Geometry: see drawing. Coordinates: mm, zero at the bounding-box minimum. Round coordinates to 2 decimals unless told otherwise and drop trailing zeros. Loops run counter-clockwise (first coordinate to the right, second up) from the corner with the lowest first, then second, coordinate; pieces in that order, holes last. Notation, with made-up numbers: M 45.5,-31 L 94.5,-31 A20 ccw 94.5,-10 Z; hole C -25,-13.5 d6. An arc over 180 degrees is marked long. Answer as a JSON object with one key per item and string values.
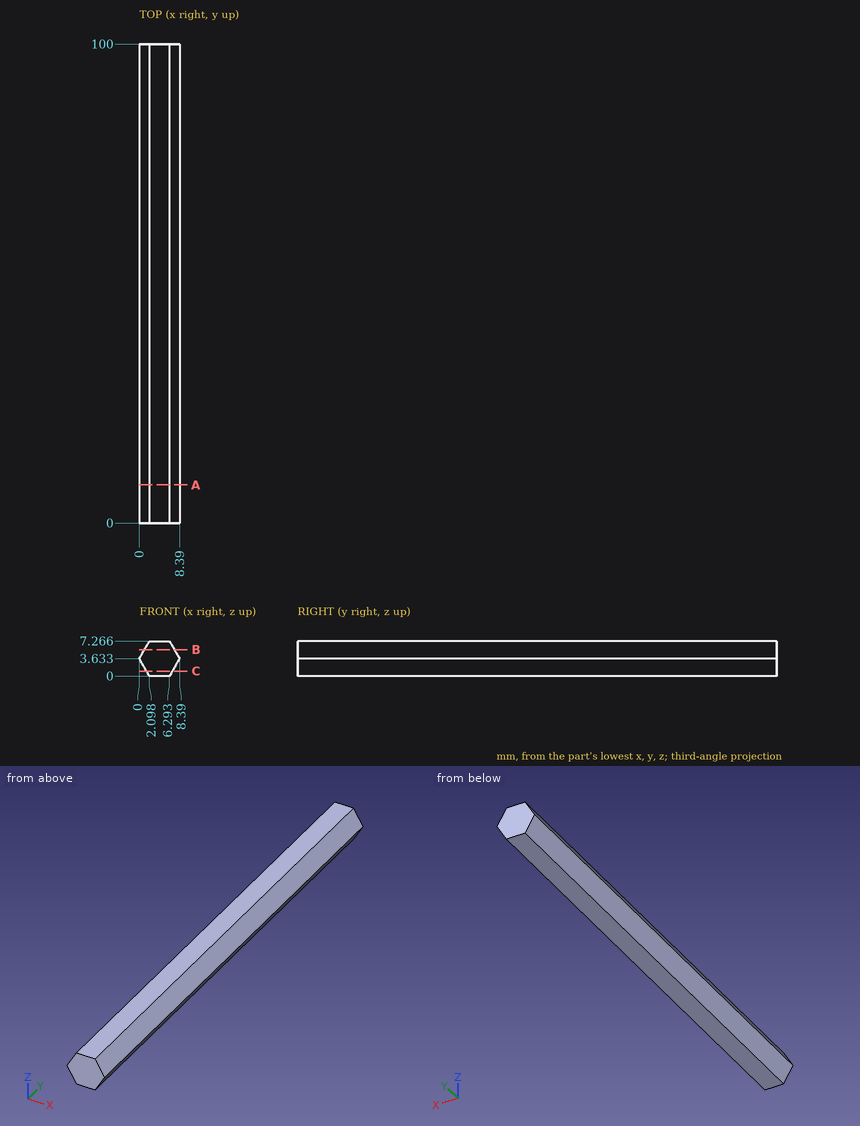
1) Pin query (flat end, axial travel): P1, Ø1, axis at y = 19.5, z = 1, coming from the -X side. Return the tip coordinate at first contact, or that it passes through.
Results:
{"P1": "x = 1.23"}
2) Section query C-C (z = 1). Return the cut outline in (x, y).
Results:
{"outline": "M 1.52,0 L 6.87,0 L 6.87,100 L 1.52,100 Z"}
3) Ray query, line 1 (X direction, y = 81, z = 4.75) (1 decimal); line 2 (X direction, y = 73.5, z = 6.25); line 3 (Z direction, x = 0.75, y = 72.5) (1 decimal). Return the intervals inside material, ascending.
Results:
{"line 1": "0.6 to 7.7", "line 2": "1.51 to 6.88", "line 3": "2.3 to 4.9"}
4) Section query B-B (z = 5.5). Return the cut outline in (x, y).
Results:
{"outline": "M 1.08,0 L 7.31,0 L 7.31,100 L 1.08,100 Z"}
5) Section query A-A (y = 8). Return the cut outline in (x, z) (1 decimal).
Results:
{"outline": "M 0,3.6 L 2.1,0 L 6.3,0 L 8.4,3.6 L 6.3,7.3 L 2.1,7.3 Z"}
